from build123d import *

# Parameters (mm, degrees)
EXTRUDE1_START = -35
SKETCH2_R      = 19.5
SKETCH2_R_2    = 19
EXTRUDE1_DEPTH = 35


with BuildPart() as part:
    # Sketch1 → Revolve1 (revolve)
    with BuildSketch(Plane(origin=(0, 0, 0), x_dir=(1, 0, 0), z_dir=(0, 1, 0))):
        Polygon((-72.838876034, 0), (-76.174491921, -3.812132442), (-76.174491921, -7.812132442), (-75.674491921, -7.812132442), (-75.674491921, -4), (-72.174491921, 0), align=None)
    revolve(axis=Axis((-57.174491921, 0, 0), (0, 0, 1)))

    # Sketch2 → Extrude1 (add)
    with BuildSketch(Plane(origin=(0, 0, 0), x_dir=(-1, 0, 0), z_dir=(0, 0, -1)).offset(EXTRUDE1_START)):
        with Locations((57.174491921, 0)):
            Circle(SKETCH2_R)
        with Locations((57.174491921, 0)):
            Circle(SKETCH2_R_2, mode=Mode.SUBTRACT)
    extrude(amount=EXTRUDE1_DEPTH)


solid = part.part
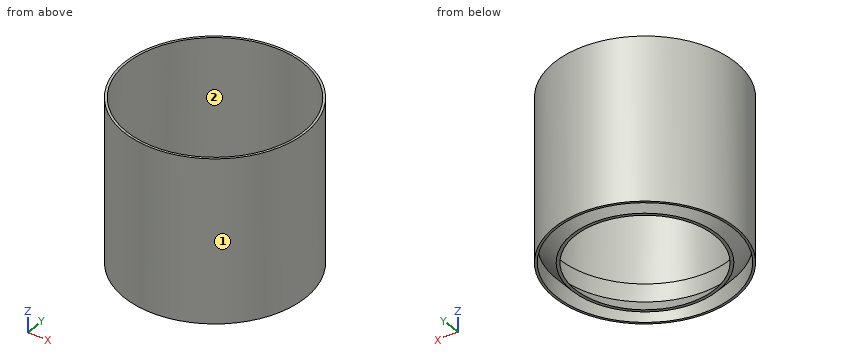
Work out the finished part from the listing and answer in its coordinate system (mm). Face numbers are marked on the shaded views. Give positions to 0.01 mm unless a question says otherwise; leave off trailing zeros. Loops run counter-clockwise (first coordinate to the right, second up) from the corner with the lowest first, then second, coordinate; pieces in that order, holes last. Notation, with made-up numbers: (-36.75, -18.75) - (-2.75, -18.75) arc R14 ccw to (-2.75, -4.75) - close; hole circle Ø9 at (72, 7). An arc over 180 degrees is marked (long way). Answer in a Markdown table with one row per item.
(1) For a pull along Y with two mould halves and no side action, classify the marked faces 1 and 2 as pulls with the +Y half, pulls with the -Y half, needs draft (parallel to the pull), parting line crosses it, or undercut.
Results list:
| item | result |
|---|---|
| face 1 | parting line crosses it |
| face 2 | undercut |
(2) Consider L1, parallel to Y at x = -47, z = 25.5; L2, parallel to Y at x = -59.5, z = 9.5; L3, parallel to X at y = -1, z = 18.5. Determine where each line is inside the solid, lowest interval first. Write a range as [from, to].
Results list:
| item | result |
|---|---|
| L1 | y = [-16.64, -16.05], [16.05, 16.64] |
| L2 | y = [-19.36, -18.86], [18.86, 19.36] |
| L3 | x = [-76.65, -76.15], [-38.2, -37.7] |
(3) Section B-B (z = 15) is taken. Give the vertices of the cut face in (x, y).
Results list:
| item | result |
|---|---|
| outline | circle Ø39 at (-57.17, 0); hole circle Ø38 at (-57.17, 0) |
(4) Flat-ended cylindrical pins translate along their axes: pin 1 Ø1 at (y, z) = (10.5, 8.5) entering from +X; pin 2 Ø12 at (y, z) = (-10, 18.5) entering from +X; pin 3 Ø6 at (x, z) = (-43, 24) entering from +Y. Find the tip coordinate at first contact, or state that the pin passes through.
Results list:
| item | result |
|---|---|
| pin 1 | stops at x = -40.43 |
| pin 2 | stops at x = -38.09 |
| pin 3 | stops at y = 15.98 |
(5) Section A-A (y = 0) is taken. Give the vertices of the cut face in (x, z).
Results list:
| item | result |
|---|---|
| outline | (-76.67, 0) - (-76.17, 0) - (-76.17, 3.81) - (-72.84, 0) - (-72.17, 0) - (-75.67, 4) - (-75.67, 7.81) - (-76.17, 7.81) - (-76.17, 35) - (-76.67, 35) - close; (-42.17, 0) - (-41.51, 0) - (-38.17, 3.81) - (-38.17, 0) - (-37.67, 0) - (-37.67, 35) - (-38.17, 35) - (-38.17, 7.81) - (-38.67, 7.81) - (-38.67, 4) - close |
